Verification items for the finished model (mm, model axes). Coordinates: 2 decimals unless noted, no trailing zeros. Write each loop counter-clockwise with the first axis right and the second up, starting at its lowest first coordinate (ties: lowest second). Pieces come first, ordered by that corner, then holes. Notation, with made-up numbers: M 23.25,-18 L 65.25,-18 A26 ccw 65.25,14 Z; hole C -14.5,-29 d11. An arc over 180 degrees is marked long. One line per item, written item: value.
```python
from build123d import *

# Parameters (mm, degrees)
BOSS_EXTRUDE1_DEPTH = 914.4
BOSS_EXTRUDE2_DEPTH = 381


with BuildPart() as part:
    # Sketch1 → Boss-Extrude1 (new body, symmetric)
    with BuildSketch(Plane(origin=(0, 0, 0), x_dir=(0, 0, -1), z_dir=(1, 0, 0))):
        Polygon((-381, 0), (381, 0), (381, -31.75), (349.25, -31.75), (349.25, -27.178), (376.428, -27.178), (376.428, -4.572), (-376.428, -4.572), (-376.428, -27.178), (-349.25, -27.178), (-349.25, -31.75), (-381, -31.75), align=None)
    extrude(amount=BOSS_EXTRUDE1_DEPTH, both=True)

    # Sketch2 → Boss-Extrude2 (add, symmetric)
    with BuildSketch(Plane.XY):
        Polygon((-914.4, 0), (-914.4, -31.75), (-882.65, -31.75), (-882.65, -27.178), (-909.828, -27.178), (-909.828, 0), align=None)
        Polygon((909.828, 0), (914.4, 0), (914.4, -31.75), (882.65, -31.75), (882.65, -27.178), (909.828, -27.178), align=None)
    extrude(amount=BOSS_EXTRUDE2_DEPTH, both=True)


solid = part.part
```
Item 1: Cross-section at C-C, the plane z = 163.5. Enter the section's corners in (x, y).
The answers:
outline: M -914.4,-31.75 L -882.65,-31.75 L -882.65,-27.18 L -909.83,-27.18 L -909.83,-4.57 L 909.83,-4.57 L 909.83,-27.18 L 882.65,-27.18 L 882.65,-31.75 L 914.4,-31.75 L 914.4,0 L -914.4,0 Z
Item 2: Draft check along X on faces 1 (the face through (13, -4.572, -5)), 2 (the face through (13, 0, 5)), 3 (the face through (-4, -27.178, 364)), 4 (the face through (914.4, -16, -5)). Enter one of: released by +X, released by -X, zero draft, split by the parting line, or undercut.
The answers:
face 1: undercut
face 2: zero draft
face 3: undercut
face 4: released by +X
Item 3: Go/stop test with a flat-tipped pin: P1, Ø4, axis at x = 391, z = 60, coming from the -Y side. Record where the tip stops, or that it passes through.
The answers:
P1: stops at y = -4.57
Item 4: Cross-section at B-B, the plane x = -519.5. Enter the section's corners in (y, z).
The answers:
outline: M -31.75,-381 L 0,-381 L 0,381 L -31.75,381 L -31.75,349.25 L -27.18,349.25 L -27.18,376.43 L -4.57,376.43 L -4.57,-376.43 L -27.18,-376.43 L -27.18,-349.25 L -31.75,-349.25 Z
Item 5: Cross-section at A-A, the plane y = -11. Enter the section's corners in (x, z).
The answers:
outline: M -914.4,-381 L 914.4,-381 L 914.4,381 L -914.4,381 Z; hole M -909.83,-376.43 L 909.83,-376.43 L 909.83,376.43 L -909.83,376.43 Z
Item 6: Scan lines: line 1 (Z direction, x = -763.5, y = -21); line 2 (X direction, y = -18, z = -58); line 3 (Y direction, x = 384, z = -137). Record each from-to range of solid material in increasing order.
The answers:
line 1: z = -381 to -376.43, 376.43 to 381
line 2: x = -914.4 to -909.83, 909.83 to 914.4
line 3: y = -4.57 to 0
